CAD build for the part. Positions are in the model's coordinates, mm. Face numbers are marked on the shaded views. A direction names the side the tool comes from. Coordinates: 2 decimals unless noted, no trailing zeros. Loops run counter-clockwise (first coordinate to the right, second up) from the corner with the lowest first, then second, coordinate; pieces in that order, holes last. Notation, with made-up numbers: (-2.5, -30) -> (35.5, -30) arc R33 ccw to (35.5, 3) -> close; hole circle Ø10 at (78, 22.25). An arc over 180 degrees is marked (long way). Return JSON: item names as keys, results as strings. Group by question number.
(1) Saw through at A-A on x = 0. Write the cut outline in (y, z).
(2) Saw through at D-D on y = 29. Write the cut outline in (x, z), then the cut area to 3 significant figures.
(3) Saw through at C-C on y = 74. Write the cut outline in (x, z).
(4) Saw through at B-B on z = 0. Write the cut outline in (x, y), then the cut area to 3 significant figures.
(5) Tool access for the marked faces 1, 2 and 3: list every direction of +Z, -Z, +X, -X, +Y, -Y with a clear straight run to the whole face (end or side of a thin tool).
(6) Probe L1, parallel to Y at x = -18.5, z = -1.5; L2, parallel to X at y = 74.5, z = 5 (3 decimals); L3, parallel to Y at x = 3, z = -2. List the from-to ranges inside material, lowest first.
(7) Flat gauge pins, fed straight in: pin 1 Ø1 at (y, z) = (38.5, 15.5) entering from -X; pin 2 Ø5 at (y, z) = (50, -1) entering from -X; pin 3 Ø12 at (y, z) = (67, -3.5) entering from +X. Where does each tip first touch, or does it go through?
```python
from build123d import *

# Parameters (mm, degrees)
SKETCH1_R           = 21
BOSS_EXTRUDE1_DEPTH = 66.5
SKETCH3_R           = 8.75
BOSS_EXTRUDE2_DEPTH = 5
FILLET1_R           = 2
SKETCH4_R           = 8
BOSS_EXTRUDE3_DEPTH = 42
SKETCH5_R           = 7.25
BOSS_EXTRUDE4_DEPTH = 5
FILLET2_R           = 1
SKETCH6_R           = 2.5
BOSS_EXTRUDE5_DEPTH = 7
FILLET3_R           = 0.5


with BuildPart() as part:
    # Sketch1 → Boss-Extrude1 (new body)
    with BuildSketch(Plane(origin=(0, 0, 0), x_dir=(1, 0, 0), z_dir=(0, 1, 0))):
        with Locations(Location((0, 0, 0), (0, 0, 270))):
            Circle(SKETCH1_R)
    extrude(amount=BOSS_EXTRUDE1_DEPTH)

    # Sketch3 → Boss-Extrude2 (add)
    with BuildSketch(Plane(origin=(0, 66.5, 0), x_dir=(1, 0, 0), z_dir=(0, 1, 0))):
        with Locations(Location((0, 0, 0), (0, 0, 270))):
            Circle(SKETCH3_R)
    extrude(amount=BOSS_EXTRUDE2_DEPTH)

    # Fillet1
    fillet1_edges = [part.edges().sort_by_distance(p)[0] for p in [
        (0, 66.5, -21),
    ]]
    fillet(fillet1_edges, radius=FILLET1_R)

    # Sketch4 → Boss-Extrude3 (add)
    with BuildSketch(Plane(origin=(0, 71.5, 0), x_dir=(1, 0, 0), z_dir=(0, 1, 0))):
        with Locations(Location((0, 0, 0), (0, 0, 90))):
            Circle(SKETCH4_R)
    extrude(amount=BOSS_EXTRUDE3_DEPTH)

    # Sketch5 → Boss-Extrude4 (add)
    with BuildSketch(Plane.XZ):
        with Locations(Location((0, 0, 0), (0, 0, 270))):
            Circle(SKETCH5_R)
    extrude(amount=BOSS_EXTRUDE4_DEPTH)

    # Fillet2
    # the kernel refuses this fillet: 1 mm, written as the material it takes off along each edge
    with BuildSketch(Plane(origin=(0, -5, 0), x_dir=(0, 0, -1), z_dir=(-1, 0, 0))) as fillet2_piece_1:
        with BuildLine():
            CenterArc((7.25 - FILLET2_R, -FILLET2_R), FILLET2_R, 0, 90)
            Line((7.25 - FILLET2_R, 0), (7.25 - FILLET2_R, FILLET2_R * 0.02))
            Line((7.25 - FILLET2_R, FILLET2_R * 0.02), (7.25 + FILLET2_R * 0.02, FILLET2_R * 0.02))
            Line((7.25 + FILLET2_R * 0.02, FILLET2_R * 0.02), (7.25 + FILLET2_R * 0.02, -FILLET2_R))
            Line((7.25 + FILLET2_R * 0.02, -FILLET2_R), (7.25, -FILLET2_R))
        make_face()
    revolve(axis=Axis((0, -5, 0), (0, -1, 0)), mode=Mode.SUBTRACT)
    with BuildSketch(Plane(origin=(0, 71.5, 0), x_dir=(0, 0, 1), z_dir=(-1, 0, 0))) as fillet2_piece_2:
        with BuildLine():
            CenterArc((7.75, -0.968245837), FILLET2_R, 0, 75.522487814)
            Line((8, 0), (8.005, 0.019364917))
            ThreePointArc((8.005, 0.019364917), (8.375, 0.02), (8.75, 0.02))
            Line((8.75, 0.02), (8.77, 0))
            Line((8.77, 0), (8.77, -0.968245837))
            Line((8.77, -0.968245837), (8.75, -0.968245837))
        make_face()
    revolve(axis=Axis((0, 71.5, 0), (0, 1, 0)), mode=Mode.SUBTRACT)

    # Sketch6 → Boss-Extrude5 (add)
    with BuildSketch(Plane.XZ.offset(5)):
        with Locations(Location((0, 0, 0), (0, 0, 270))):
            Circle(SKETCH6_R)
    extrude(amount=BOSS_EXTRUDE5_DEPTH)

    # Fillet3
    fillet3_edges = [part.edges().sort_by_distance(p)[0] for p in [
        (0, -12, 2.5),
    ]]
    fillet(fillet3_edges, radius=FILLET3_R)


solid = part.part
```
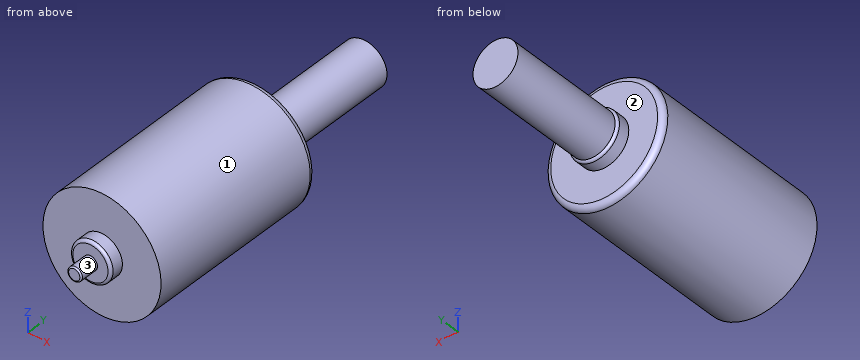
Geometry results:
{
 "1": {"outline": "(-12, -2) arc R0.5 ccw to (-11.5, -2.5) -> (-5, -2.5) -> (-5, -6.25) arc R1 ccw to (-4, -7.25) -> (0, -7.25) -> (0, -21) -> (64.5, -21) arc R2 ccw to (66.5, -19) -> (66.5, -8.75) -> (70.53, -8.75) arc R1 ccw to (71.5, -8) -> (113.5, -8) -> (113.5, 8) -> (71.5, 8) arc R1 ccw to (70.53, 8.75) -> (66.5, 8.75) -> (66.5, 19) arc R2 ccw to (64.5, 21) -> (0, 21) -> (0, 7.25) -> (-4, 7.25) arc R1 ccw to (-5, 6.25) -> (-5, 2.5) -> (-11.5, 2.5) arc R0.5 ccw to (-12, 2) -> close"},
 "2": {"outline": "circle Ø42 at (0, 0)", "area": "1,390 mm²"},
 "3": {"outline": "circle Ø16 at (0, 0)"},
 "4": {"outline": "(-21, 0) -> (-7.25, 0) -> (-7.25, -4) arc R1 ccw to (-6.25, -5) -> (-2.5, -5) -> (-2.5, -11.5) arc R0.5 ccw to (-2, -12) -> (2, -12) arc R0.5 ccw to (2.5, -11.5) -> (2.5, -5) -> (6.25, -5) arc R1 ccw to (7.25, -4) -> (7.25, 0) -> (21, 0) -> (21, 64.5) arc R2 ccw to (19, 66.5) -> (8.75, 66.5) -> (8.75, 70.53) arc R1 ccw to (8, 71.5) -> (8, 113.5) -> (-8, 113.5) -> (-8, 71.5) arc R1 ccw to (-8.75, 70.53) -> (-8.75, 66.5) -> (-19, 66.5) arc R2 ccw to (-21, 64.5) -> close", "area": "3,660 mm²"},
 "5": {"face 1": "+Y, -Y", "face 2": "+Y", "face 3": "-Y"},
 "6": {"L1": "0 to 66.5", "L2": "-6.245 to 6.245", "L3": "-5 to 113.5"},
 "7": {"pin 1": "x = -14.7", "pin 2": "x = -21", "pin 3": "x = 21"}
}
